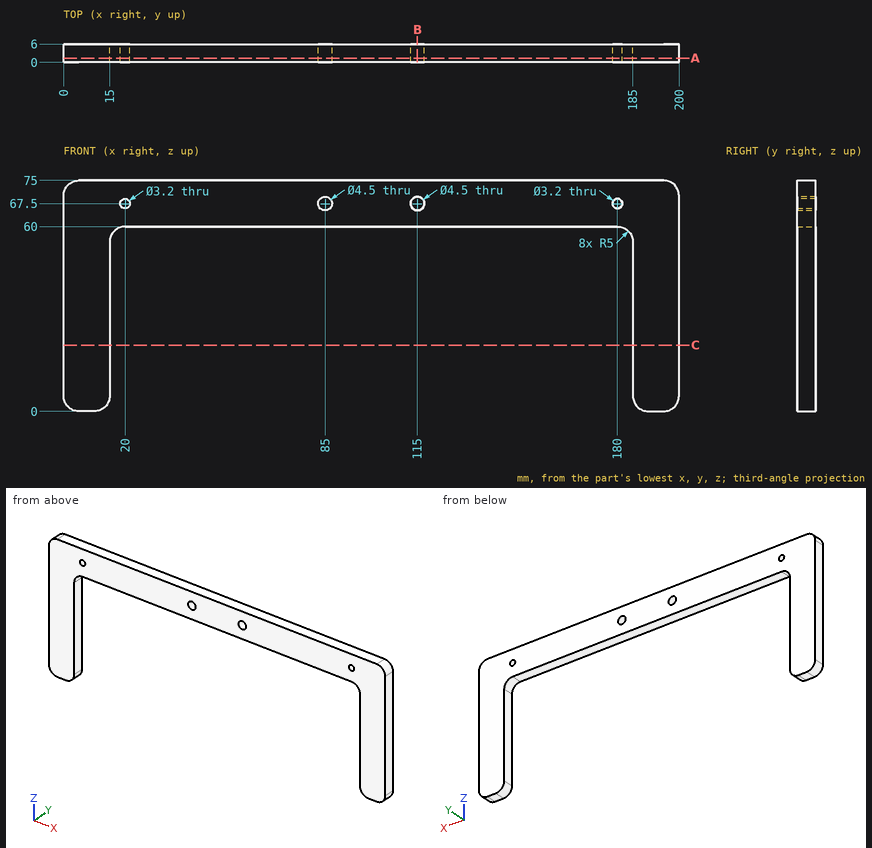
Design review of the part shown in the three views and the two pictorial views. Dimensions are in mm from the part's minimum x, y and z. Give positions to 0.01 mm unless a question says otherwise; leave off trailing zeros. Loops run counter-clockwise (first coordinate to the right, second up) from the corner with the lowest first, then second, coordinate; pieces in that order, holes last. Notation, with made-up numbers: M 79.25,-12 L 135.25,-12 A19 ccw 135.25,22 Z; hole C -36.5,42.25 d10. An arc over 180 degrees is marked long. Answer as a JSON object with one key per item and string values.
Item 1: For P1, Ø6, axis at x = 171, z = 56, coming from the -Y side, flat-tipped, find the tip position at first contact; note if it passes through.
Output values:
{"P1": "passes through"}
Item 2: We need section A-A (y = 1.4). State the section outline as (x, z) points.
Output values:
{"outline": "M 0,5 A5 ccw 5,0 L 10,0 A5 ccw 15,5 L 15,55 A5 cw 20,60 L 180,60 A5 cw 185,55 L 185,5 A5 ccw 190,0 L 195,0 A5 ccw 200,5 L 200,70 A5 ccw 195,75 L 5,75 A5 ccw 0,70 Z; hole C 20,67.5 d3.2; hole C 85,67.5 d4.5; hole C 115,67.5 d4.5; hole C 180,67.5 d3.2"}
Item 3: Wall thickness on line 1 along X through (y, z) = (2, 67.5); line 2 along X through (y, z) = (2.6, 25.5); line 3 along X through (y, z) = (5.2, 68.5): over which ranges is each line inside the solid? List them lowest first.
Output values:
{"line 1": "x = 0 to 18.4, 21.6 to 82.75, 87.25 to 112.75, 117.25 to 178.4, 181.6 to 200", "line 2": "x = 0 to 15, 185 to 200", "line 3": "x = 0 to 18.75, 21.25 to 82.98, 87.02 to 112.98, 117.02 to 178.75, 181.25 to 200"}
Item 4: We need section B-B (x = 115). State the section outline as (y, z) points.
Output values:
{"outline": "M 0,60 L 6,60 L 6,65.25 L 0,65.25 Z; M 0,69.75 L 6,69.75 L 6,75 L 0,75 Z"}
Item 5: We need section C-C (z = 21.5). State the section outline as (x, y) points, and give its area (3 significant figures).
Output values:
{"outline": "M 0,0 L 15,0 L 15,6 L 0,6 Z; M 185,0 L 200,0 L 200,6 L 185,6 Z", "area": "180 mm2"}
